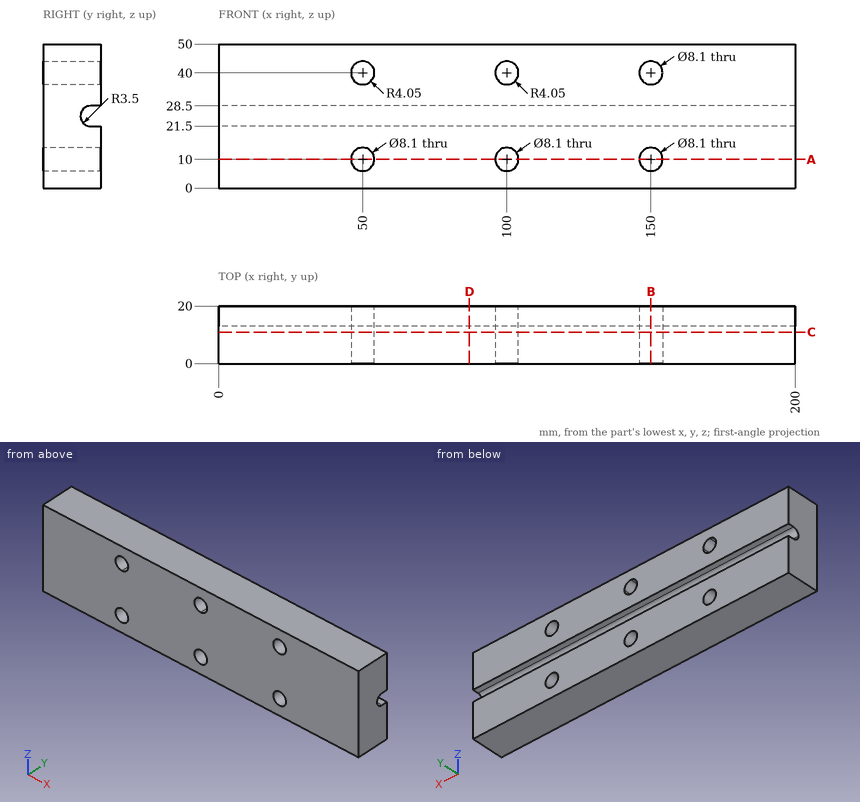
Geometry check sheet. Reference: drawing and pictorial views, mm from the part's lowest x, y, z. Give positions to 0.01 mm unless a question says otherwise; leave off trailing zeros. Write each loop counter-clockwise with the first axis right and the second up, starting at its lowest first coordinate (ties: lowest second). Pieces come first, ordered by that corner, then holes. Notation, with made-up numbers: (85, 22) - (136, 22) arc R24 cw to (136, 57) - close; hole circle Ø2 at (9, 79). An arc over 180 degrees is marked (long way). Use a Markdown table: item, result.
Q1. Section check D-D, the plane x = 87. Enter the section's corners in (y, z).
Computed:
| item | result |
|---|---|
| outline | (0, 0) - (20, 0) - (20, 21.5) - (16.5, 21.5) arc R3.5 cw to (16.5, 28.5) - (20, 28.5) - (20, 50) - (0, 50) - close |
Q2. Section check C-C, the plane y = 11. Enter the section's corners in (x, z).
Computed:
| item | result |
|---|---|
| outline | (0, 0) - (200, 0) - (200, 50) - (0, 50) - close; hole circle Ø8.1 at (50, 10); hole circle Ø8.1 at (50, 40); hole circle Ø8.1 at (100, 10); hole circle Ø8.1 at (100, 40); hole circle Ø8.1 at (150, 10); hole circle Ø8.1 at (150, 40) |
Q3. Section check B-B, the plane x = 150. Enter the section's corners in (y, z).
Computed:
| item | result |
|---|---|
| outline | (0, 0) - (20, 0) - (20, 5.95) - (0, 5.95) - close; (0, 14.05) - (20, 14.05) - (20, 21.5) - (16.5, 21.5) arc R3.5 cw to (16.5, 28.5) - (20, 28.5) - (20, 35.95) - (0, 35.95) - close; (0, 44.05) - (20, 44.05) - (20, 50) - (0, 50) - close |
Q4. Thickness scan on L1, parallel to X at y = 11.25, z = 40; L2, parallel to Z at x = 37, y = 18.75; L3, parallel to X at y = 4.25, z = 37. Record the ranges inside material, lowest first. Write a range as [from, to].
Computed:
| item | result |
|---|---|
| L1 | x = [0, 45.95], [54.05, 95.95], [104.05, 145.95], [154.05, 200] |
| L2 | z = [0, 21.5], [28.5, 50] |
| L3 | x = [0, 47.28], [52.72, 97.28], [102.72, 147.28], [152.72, 200] |
Q5. Section check A-A, the plane z = 10. Enter the section's corners in (x, y).
Computed:
| item | result |
|---|---|
| outline | (0, 0) - (45.95, 0) - (45.95, 20) - (0, 20) - close; (54.05, 0) - (95.95, 0) - (95.95, 20) - (54.05, 20) - close; (104.05, 0) - (145.95, 0) - (145.95, 20) - (104.05, 20) - close; (154.05, 0) - (200, 0) - (200, 20) - (154.05, 20) - close |
